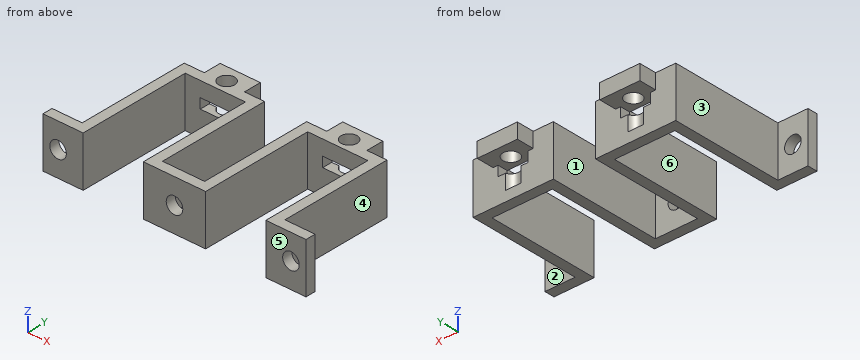
```python
from build123d import *

# Parameters (mm, degrees)
EXTRUIR_L_MINA1_DEPTH   = 10
CROQUIS2_W              = 8
CROQUIS2_H              = 3.5
SALIENTE_EXTRUIR1_DEPTH = 3
CROQUIS3_R              = 1.65
CORTAR_EXTRUIR1_DEPTH   = 40.628777422
CROQUIS4_R              = 1.6
CORTAR_EXTRUIR2_DEPTH   = 8
CROQUIS6_W              = 6
CROQUIS6_H              = 2
CORTAR_EXTRUIR3_DEPTH   = 38.238286749


with BuildPart() as part:
    # Croquis1 → Extruir-Lámina1 (new body)
    with BuildSketch(Plane.XY):
        Polygon((26.2, 0), (18.2, 0), (18.2, 22.5), (6.2, 22.5), (6.2, 0), (-6.2, 0), (-6.2, 22.5), (-18.2, 22.5), (-18.2, 0), (-26.2, 0), (-26.2, 2), (-20.2, 2), (-20.2, 24.5), (-4.2, 24.5), (-4.2, 2), (4.2, 2), (4.2, 24.5), (20.2, 24.5), (20.2, 2), (26.2, 2), align=None)
    extrude(amount=EXTRUIR_L_MINA1_DEPTH)

    # Croquis2 → Saliente-Extruir1 (add)
    with BuildSketch(Plane.XY.offset(10)):
        with Locations((-12.2, 26.25)):
            Rectangle(CROQUIS2_W, CROQUIS2_H)
    saliente_extruir1 = extrude(amount=-SALIENTE_EXTRUIR1_DEPTH)

    # Simetría1: Saliente-Extruir1 across plane
    add(saliente_extruir1.mirror(Plane(origin=(0, 0, 0), x_dir=(0, 0, 1), z_dir=(1, 0, 0))))

    # Croquis3 → Cortar-Extruir1 (cut, through all)
    with BuildSketch(Plane(origin=(0, 0, 0), x_dir=(-1, 0, 0), z_dir=(0, -1, 0))):
        with Locations(Location((0, -5, 0), (0, 0, 90))):
            Circle(CROQUIS3_R)
        with Locations(Location((23.2, -5, 0), (0, 0, 90))):
            Circle(CROQUIS3_R)
        with Locations(Location((-23.2, -5, 0), (0, 0, 90))):
            Circle(CROQUIS3_R)
    extrude(amount=-CORTAR_EXTRUIR1_DEPTH, mode=Mode.SUBTRACT)

    # Croquis4 → Cortar-Extruir2 (cut)
    with BuildSketch(Plane.XY.offset(10)):
        with Locations((-12.2, 25)):
            Circle(CROQUIS4_R)
    cortar_extruir2 = extrude(amount=-CORTAR_EXTRUIR2_DEPTH, mode=Mode.SUBTRACT)

    # Croquis6 → Cortar-Extruir3 (cut, through all)
    with BuildSketch(Plane(origin=(0, 24.5, 0), x_dir=(1, 0, 0), z_dir=(0, 1, 0))):
        with Locations((-12.2, -6)):
            Rectangle(CROQUIS6_W, CROQUIS6_H)
    cortar_extruir3 = extrude(amount=-CORTAR_EXTRUIR3_DEPTH, mode=Mode.SUBTRACT)

    # Simetría2: Cortar-Extruir2, Cortar-Extruir3 across plane
    add(cortar_extruir2.mirror(Plane(origin=(0, 0, 0), x_dir=(0, 0, 1), z_dir=(1, 0, 0))), mode=Mode.SUBTRACT)
    add(cortar_extruir3.mirror(Plane(origin=(0, 0, 0), x_dir=(0, 0, 1), z_dir=(1, 0, 0))), mode=Mode.SUBTRACT)


solid = part.part
```
Read the model definition and answer for the solid it produces. Units are mm, in the model's axes. Face numbers are marked on the shaded views. A direction names the side the tool comes from. Give positions to 0.01 mm unless a question says otherwise; leave off trailing zeros. Order: outer loops, then holes, each group sorted by start corner. A loop starts at its lowest first (then second) coordinate and runs counter-clockwise, first axis right, second up. Notation, with made-up numbers: (52, 38.5) -> (84, 38.5) arc R13 ccw to (84, 62.5) -> close; hole circle Ø2 at (-1.75, 39.5). An arc over 180 degrees is marked (long way). One line per item, written item: value. Start each with the question number.
(1) For a pull along X with two mould halves and no side action, classify the marked faces 4, 5 and 6 as released by +X, released by -X, zero draft, split by the parting line, or undercut.
(2) The part is cut by section C-C (y = 25). Determine the outline of the cut face in (x, z).
(3) The part is cut by section D-D (z = 1). Determine the outline of the cut face in (x, y).
(4) Flat-ended cylindrical pins translate along their axes: P1, Ø3, axis at x = -1.5, y = 7.5, coming from the -Z side; P2, Ø3, axis at y = 9.5, z = 6, coming from the -X side; P3, Ø2, axis at x = 11, y = 24, coming from the +Z side; P4, Ø6, axis at y = 23, z = 4.5, coming from the +X side. Find the tip coordinate at first contact, or state that the pin passes through.
(5) Straight lines are drawn through the part: L1, parallel to X at y = 18.5, z = 3.75; L2, parallel to X at y = 0.95, z = 5; L3, parallel to Y at x = -12.2, z = 8.55. For each, find the intervals that lie inside material, in ascending order.
(6) The part is cut by section B-B (x = 10). Determine the outline of the cut face in (y, z).
(7) The part is cut by section A-A (y = 12.75). Determine the outline of the cut face in (x, z), and give its area (3 significant figures).
(8) A tool of negligible diameter and unlimited length cuts with its end or side. For the marked faces 1, 2 and 3, from which of +Z, -Z, +X, -X, +Y, -Y can it reach the whole face along a straight path? Write none if from no direction.
Taken from the geometry:
1. face 4: released by +X
1. face 5: zero draft
1. face 6: undercut
2. outline: (-16.2, 7) -> (-13.8, 7) -> (-13.8, 10) -> (-16.2, 10) -> close; (-10.6, 7) -> (-8.2, 7) -> (-8.2, 10) -> (-10.6, 10) -> close; (8.2, 7) -> (10.6, 7) -> (10.6, 10) -> (8.2, 10) -> close; (13.8, 7) -> (16.2, 7) -> (16.2, 10) -> (13.8, 10) -> close
3. outline: (-26.2, 0) -> (-18.2, 0) -> (-18.2, 22.5) -> (-6.2, 22.5) -> (-6.2, 0) -> (6.2, 0) -> (6.2, 22.5) -> (18.2, 22.5) -> (18.2, 0) -> (26.2, 0) -> (26.2, 2) -> (20.2, 2) -> (20.2, 24.5) -> (4.2, 24.5) -> (4.2, 2) -> (-4.2, 2) -> (-4.2, 24.5) -> (-20.2, 24.5) -> (-20.2, 2) -> (-26.2, 2) -> close
4. P1: through
4. P2: x = -20.2
4. P3: z = 10
4. P4: x = 20.2
5. L1: -20.2 to -18.2, -6.2 to -4.2, 4.2 to 6.2, 18.2 to 20.2
5. L2: -26.2 to -24.85, -21.55 to -18.2, -6.2 to -1.65, 1.65 to 6.2, 18.2 to 21.55, 24.85 to 26.2
5. L3: 22.5 to 23.4, 26.6 to 28
6. outline: (22.5, 0) -> (24.5, 0) -> (24.5, 5) -> (22.5, 5) -> close; (22.5, 7) -> (28, 7) -> (28, 10) -> (22.5, 10) -> close
7. outline: (-20.2, 0) -> (-18.2, 0) -> (-18.2, 10) -> (-20.2, 10) -> close; (-6.2, 0) -> (-4.2, 0) -> (-4.2, 10) -> (-6.2, 10) -> close; (4.2, 0) -> (6.2, 0) -> (6.2, 10) -> (4.2, 10) -> close; (18.2, 0) -> (20.2, 0) -> (20.2, 10) -> (18.2, 10) -> close
7. area: 80.0 mm^2
8. face 1: +Z, -Z, +Y
8. face 2: +Z, -Z, +X, +Y
8. face 3: +Z, -Z, -X, +Y
